Design review of the part built by this model. Coordinates are the model's own, in mm. Coordinates: 2 decimals unless noted, no trailing zeros. Order: outer loops, then holes, each group sorted by start corner. A loop starts at its lowest first (then second) coordinate and runs counter-clockwise, first axis right, second up. Notation, with made-up numbers: M 86,-10 L 127,-10 A24 cw 127,1 Z; hole C 43,52.5 d9. An arc over 180 degrees is marked long. Answer in a Markdown table with one row per item.
from build123d import *

# Parameters (mm, degrees)
ESQUISSE1_W               = 100
ESQUISSE1_H               = 180
BOSS_EXTRU_1_DEPTH        = 10
M14_CLEARANCE_HOLE1_D     = 15.5
M14_CLEARANCE_HOLE1_DEPTH = 10
FILLET1_R                 = 1


with BuildPart() as part:
    # Esquisse1 → Boss.-Extru.1 (new body)
    with BuildSketch(Plane.XY):
        Rectangle(ESQUISSE1_W, ESQUISSE1_H)
    extrude(amount=BOSS_EXTRU_1_DEPTH)

    # M14 Clearance Hole1
    with Locations(Plane.XY.offset(10)):
        with Locations((0, 70), (0, -70), (60, -70), (60, 70)):
            Hole(M14_CLEARANCE_HOLE1_D / 2, depth=M14_CLEARANCE_HOLE1_DEPTH)

    # Fillet1
    fillet1_edges = [part.edges().sort_by_distance(p)[0] for p in [
        (-50, 0, 10),
        (50, 0, 10),
        (-50, 0, 0),
        (50, 0, 0),
    ]]
    fillet(fillet1_edges, radius=FILLET1_R)


solid = part.part
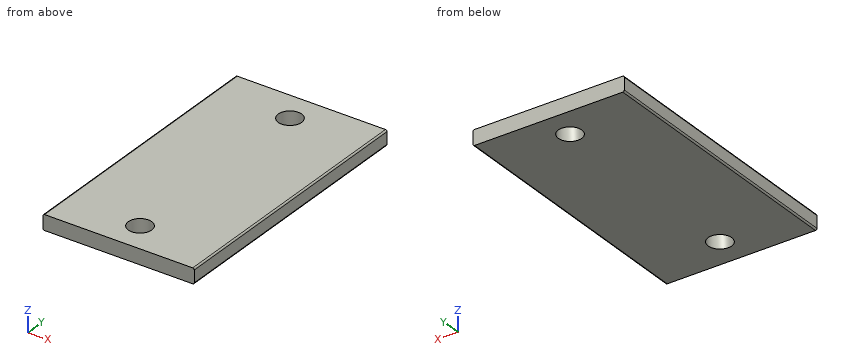
(1) For line 1 along Y through (x, z) = (0, 7.75); line 2 along X through (y, z) = (66.5, 8.5); line 3 along Y through (x, z) = (4, 6.75), list the stretches that pass through material, from the lowest coordinate up. Write a range as from..to.
Return value:
| item | result |
|---|---|
| line 1 | y = -90..-77.75, -62.25..62.25, 77.75..90 |
| line 2 | x = -50..-6.91, 6.91..50 |
| line 3 | y = -90..-76.64, -63.36..63.36, 76.64..90 |
(2) Insertion check: pin 1 Ø12.5 at (x, y) = (0, 70) entering from +Z. The pin has a flat end and moves straight along its axis. Give the tip position at first contact, or say it passes through.
Return value:
| item | result |
|---|---|
| pin 1 | passes through |
(3) Add section B-B, the plane y = -70. Give the boundary of the cut face in (x, z).
Return value:
| item | result |
|---|---|
| outline | M -50,1 A1 ccw -49,0 L -7.75,0 L -7.75,10 L -49,10 A1 ccw -50,9 Z; M 7.75,0 L 49,0 A1 ccw 50,1 L 50,9 A1 ccw 49,10 L 7.75,10 Z |
(4) Add section C-C, the plane z = 5.5. Give the boundary of the cut face in (x, y), and give its area (3 significant figures).
Return value:
| item | result |
|---|---|
| outline | M -50,-90 L 50,-90 L 50,90 L -50,90 Z; hole C 0,-70 d15.5; hole C 0,70 d15.5 |
| area | 17,600 mm2 |
(5) Add section A-A, the plane x = 0. Give the boundary of the cut face in (y, z).
Return value:
| item | result |
|---|---|
| outline | M -90,0 L -77.75,0 L -77.75,10 L -90,10 Z; M -62.25,0 L 62.25,0 L 62.25,10 L -62.25,10 Z; M 77.75,0 L 90,0 L 90,10 L 77.75,10 Z |
